```python
from build123d import *

# Parameters (mm, degrees)
F0_W     = 19.05
F0_H     = 152.4
F1_DEPTH = 2.9718
F2_R     = 6.35
F3_R     = 2.8575
F4_DEPTH = 25.4
F5_W     = 50.8
F5_H     = 50.8
F6_DEPTH = 2.9718
F7_R     = 5.08


with BuildPart() as f1:
    # F0 (on Top) → F1 (new body)
    with BuildSketch(Plane.XY):
        Rectangle(F0_W, F0_H)
    extrude(amount=F1_DEPTH)

    # F2
    f2_edges = [f1.edges().sort_by_distance(p)[0] for p in [
        (9.525, -76.2, 1.4859),
        (-9.525, -76.2, 1.4859),
    ]]
    fillet(f2_edges, radius=F2_R)

    # F3 (on face) → F4 (cut)
    with BuildSketch(Plane.XY.offset(2.9718)):
        with Locations((0, -66.675)):
            Circle(F3_R)
    extrude(amount=-F4_DEPTH, mode=Mode.SUBTRACT)

    # F5 (on face) → F6 (join)
    with BuildSketch(Plane.XY.offset(2.9718)):
        with Locations((0, 50.8)):
            Rectangle(F5_W, F5_H)
    extrude(amount=-F6_DEPTH)

    # F7
    f7_edges = [f1.edges().sort_by_distance(p)[0] for p in [
        (9.525, 25.4, 1.4859),
        (25.4, 25.4, 1.4859),
        (-9.525, 25.4, 1.4859),
        (-25.4, 25.4, 1.4859),
        (25.4, 76.2, 1.4859),
        (-25.4, 76.2, 1.4859),
    ]]
    fillet(f7_edges, radius=F7_R)


solid = f1.part
```
Verification items for the finished model (mm, model axes). A direction names the side the tool comes from. Round coordinates to 2 decimals unless told otherwise and drop trailing zeros. Order: outer loops, then holes, each group sorted by start corner. A loop starts at its lowest first (then second) coordinate and runs counter-clockwise, first axis right, second up.
1) Cross-section at A-A, the plane x = 0. Record the cut outline in (y, z).
Geometry says:
outline: (-76.2, 0) - (-69.53, 0) - (-69.53, 2.97) - (-76.2, 2.97) - close; (-63.82, 0) - (76.2, 0) - (76.2, 2.97) - (-63.82, 2.97) - close
2) Cross-section at D-D, the plane x = 12. Record the cut outline in (y, z), plus the area to 3 significant figures.
Geometry says:
outline: (24.68, 0) - (76.2, 0) - (76.2, 2.97) - (24.68, 2.97) - close
area: 153 mm2
3) Tool access check on faces 4 (the flat face through (25.4, 51, 2)), 5 (the flat face through (17, 25.4, 2)), 6 (the flat face through (-9.525, -25, 1)). Record the directions out of +Z, -Z, +X, -X, +Y, -Y that give a thin tool (end or side, any length) a straight path to the whole face; none if there is none.
Geometry says:
face 4: +Z, -Z, +X, +Y, -Y
face 5: +Z, -Z, +X, -Y
face 6: +Z, -Z, -X, -Y
4) Material ranges on line 1 (Y direction, x = 0, z = 0.6); line 2 (Y direction, x = -20, z = 2.25); line 3 (X direction, y = -57, z = 1.8) (3 decimals), recorded low to high.
Geometry says:
line 1: y = -76.2 to -69.53, -63.82 to 76.2
line 2: y = 25.4 to 76.2
line 3: x = -9.525 to 9.525
5) Depth check by flat-ended pin: pin 1 (1.5 mm diameter, centred on x = 19, z = 1, fed in from -Y); pin 2 (1 mm diameter, centred on x = 11, y = -15.5, fed in from -Z); pin 3 (0.9 mm diameter, centred on y = -12, z = 2, fed in from -X) (3 decimals). Enter the tip coordinate at first touch or a pass-through.
Geometry says:
pin 1: stops at y = 25.4
pin 2: passes through
pin 3: stops at x = -9.525
6) Cross-section at C-C, the plane y = -20.5. Record the cut outline in (x, z) (3 decimals).
Geometry says:
outline: (-9.525, 0) - (9.525, 0) - (9.525, 2.972) - (-9.525, 2.972) - close
7) Draft check along Y on faces 1 (the cylindrical face through (-0.619, -69.465, 1.507)), 2 (the cylindrical face through (-23.951, 74.672, 1.465)), 3 (the cylindrical face through (-11, 23.9, 1.5)). Enter one of: +Y half, -Y half, draft (parallel to the pull), parting line (faces both ways), or undercut.
Geometry says:
face 1: undercut
face 2: +Y half
face 3: -Y half
